```python
from build123d import *

# Parameters (mm, degrees)
SKETCH1_W                = 250
SKETCH1_H                = 100
BOSS_EXTRUDE1_DEPTH      = 4
SKETCH2_W                = 24
SKETCH2_H                = 4
BOSS_EXTRUDE2_DEPTH      = 4
SKETCH3_W                = 4
SKETCH3_H                = 40
SKETCH3_H_2              = 20
CUT_EXTRUDE1_DEPTH       = 5
M4_CLEARANCE_HOLE1_D     = 4.3
M4_CLEARANCE_HOLE1_DEPTH = 6
M4_CLEARANCE_HOLE1_TIP   = 1.291850331
CUT_EXTRUDE2_DEPTH       = 10
SKETCH7_W                = 13
SKETCH7_H                = 5
CUT_EXTRUDE3_DEPTH       = 10
CUT_EXTRUDE4_DEPTH       = 10


with BuildPart() as part:
    # Sketch1 → Boss-Extrude1 (new body)
    with BuildSketch(Plane.XY):
        Rectangle(SKETCH1_W, SKETCH1_H)
    extrude(amount=BOSS_EXTRUDE1_DEPTH)

    # Sketch2 → Boss-Extrude2 (add)
    with BuildSketch(Plane.XZ.offset(50)):
        with Locations((-78, 2)):
            Rectangle(SKETCH2_W, SKETCH2_H)
        with Locations((-42, 2)):
            Rectangle(SKETCH2_W, SKETCH2_H)
        with Locations((42, 2)):
            Rectangle(SKETCH2_W, SKETCH2_H)
        with Locations((78, 2)):
            Rectangle(SKETCH2_W, SKETCH2_H)
    boss_extrude2 = extrude(amount=BOSS_EXTRUDE2_DEPTH)

    # Sketch3 → Cut-Extrude1 (cut, through all)
    with BuildSketch(Plane.XY.offset(4)):
        with Locations((-8.5, 30)):
            Rectangle(SKETCH3_W, SKETCH3_H)
        with Locations((-8.5, -12)):
            Rectangle(SKETCH3_W, SKETCH3_H_2)
        with Locations((8.5, -12)):
            Rectangle(SKETCH3_W, SKETCH3_H_2)
        with Locations((8.5, 30)):
            Rectangle(SKETCH3_W, SKETCH3_H)
    extrude(amount=-CUT_EXTRUDE1_DEPTH, mode=Mode.SUBTRACT)

    # Mirror1: Boss-Extrude2 across plane
    add(boss_extrude2.mirror(Plane.ZX))

    # M4 Clearance Hole1
    with Locations(Plane.XY.offset(4)):
        with Locations((-8.5, 4), (8.5, 4)):
            Hole(M4_CLEARANCE_HOLE1_D / 2, depth=M4_CLEARANCE_HOLE1_DEPTH)
            with Locations((0, 0, -(M4_CLEARANCE_HOLE1_DEPTH + M4_CLEARANCE_HOLE1_TIP / 2))):  # 118° drill point
                Cone(0, M4_CLEARANCE_HOLE1_D / 2, M4_CLEARANCE_HOLE1_TIP, mode=Mode.SUBTRACT)

    # Sketch6 → Cut-Extrude2 (cut)
    with BuildSketch(Plane.XY.offset(4)):
        Polygon((-62.1, -50), (-57.9, -50), (-57.9, -40), (-55.5, -40), (-55.5, -39), (-56.25, -39), (-56.25, -36.5), (-57.9, -36.5), (-57.9, -33), (-62.1, -33), (-62.1, -36.5), (-63.75, -36.5), (-63.75, -39), (-64.5, -39), (-64.5, -40), (-62.1, -40), align=None)
        Polygon((57.9, -40), (57.9, -50), (62.1, -50), (62.1, -40), (64.5, -40), (64.5, -39), (63.75, -39), (63.75, -36.5), (62.1, -36.5), (62.1, -33), (57.9, -33), (57.9, -36.5), (56.25, -36.5), (56.25, -39), (55.5, -39), (55.5, -40), align=None)
        Polygon((62.1, 40), (62.1, 50), (57.9, 50), (57.9, 40), (55.5, 40), (55.5, 39), (56.25, 39), (56.25, 36.5), (57.9, 36.5), (57.9, 33), (62.1, 33), (62.1, 36.5), (63.75, 36.5), (63.75, 39), (64.5, 39), (64.5, 40), align=None)
        Polygon((-57.9, 50), (-62.1, 50), (-62.1, 40), (-64.5, 40), (-64.5, 39), (-63.75, 39), (-63.75, 36.5), (-62.1, 36.5), (-62.1, 33), (-57.9, 33), (-57.9, 36.5), (-56.25, 36.5), (-56.25, 39), (-55.5, 39), (-55.5, 40), (-57.9, 40), align=None)
    extrude(amount=-CUT_EXTRUDE2_DEPTH, mode=Mode.SUBTRACT)

    # Sketch7 → Cut-Extrude3 (cut)
    with BuildSketch(Plane.XY.offset(4)):
        with Locations((0, 47.5)):
            Rectangle(SKETCH7_W, SKETCH7_H)
    extrude(amount=-CUT_EXTRUDE3_DEPTH, mode=Mode.SUBTRACT)

    # Sketch8 → Cut-Extrude4 (cut)
    with BuildSketch(Plane.XY.offset(4)):
        Polygon((-15.5, 50), (-32.700401322, 262.698056725), (-161.835837728, 81.113354009), (-171.999440278, -88.149719236), (-15.5, -103.395123062), align=None)
    extrude(amount=-CUT_EXTRUDE4_DEPTH, mode=Mode.SUBTRACT)


solid = part.part
```
Geometry: final body of the model. Coordinates: model frame, mm. A direction names the side the tool comes from. Coordinates: 2 decimals unless noted, no trailing zeros. Order: outer loops, then holes, each group sorted by start corner. A loop starts at its lowest first (then second) coordinate and runs counter-clockwise, first axis right, second up. Notation, with made-up numbers: M 52.25,-30.5 L 69.25,-30.5 A21 ccw 69.25,4.5 Z; hole C 64,41.25 d4. An arc over 180 degrees is marked long. Answer in a Markdown table with one row per item. Add a question column.
Q1. Reachability of faces 1 (the flat face through (66, -52, 2)), 2 (the flat face through (7, -50, 2)), 3 (the flat face through (107, -50, 2)), 4 (the flat face through (107, 50, 2)), 5 (the flat face through (-6.5, 27, 2)) from +Z, -Z, +X, -X, +Y, -Y: full face, straight path, thin tool, end or side. Return the list, or none.
Q2. Section query B-B on y = 4. Return the cut outline in (x, z).
Q3. Section query A-A on x = -8.5. Return the cut outline in (y, z).
Q4. Mould query, pull axis Y, two halves, no side actions, for faces 6 (the flat face through (57.9, -35, 2)), 7 (the flat face through (0, 45, 2)), 8 (the flat face through (-10.5, -12, 2)). Classes: released by +Y, released by -Y, zero draft, split by the parting line, or undercut.
Q5. Section query C-C on y = -46. Return the cut outline in (x, z), and give its area (3 significant figures).
Q6. Contact query for flat-ended pins moving along their axis: P1, Ø1.2, axis at x = 8, z = 2.5, coming from the -Y side; P2, Ø1.5, axis at x = 7.5, y = 37.5, coming from the -Z side; P3, Ø0.5, axis at x = 63, z = 1, coming from the +Y side; P4, Ø2, axis at y = -51.5, z = 2, coming from the +X side. Output: stop coordinate, or through.
Q7. Section query D-D on z = 2.5. Count the separate pieces of the cut face and the enclosed holes in it, and give its area (3 significant figures).
Q8. Line query: L1, parallel to X at y = 22, z = 3.65; L2, parallel to X at y = 35, z = 3.1; L3, parallel to Y at x = -8.5, z = 2.15. Output: solid intervals per line, ascending.
Completed:
| question | item | result |
|---|---|---|
| 1 | face 1 | +Z, -Z, -Y |
| 1 | face 2 | +Z, -Z, -X, -Y |
| 1 | face 3 | +Z, -Z, +X, -Y |
| 1 | face 4 | +Z, -Z, +X, +Y |
| 1 | face 5 | +Z, -Z, +Y |
| 2 | outline | M -15.5,0 L -10.65,0 L -10.65,4 L -15.5,4 Z; M -6.35,0 L 6.35,0 L 6.35,4 L -6.35,4 Z; M 10.65,0 L 125,0 L 125,4 L 10.65,4 Z |
| 3 | outline | M -50,0 L -22,0 L -22,4 L -50,4 Z; M -2,0 L 1.85,0 L 1.85,4 L -2,4 Z; M 6.15,0 L 10,0 L 10,4 L 6.15,4 Z |
| 4 | face 6 | zero draft |
| 4 | face 7 | released by +Y |
| 4 | face 8 | undercut |
| 5 | outline | M -15.5,0 L 57.9,0 L 57.9,4 L -15.5,4 Z; M 62.1,0 L 125,0 L 125,4 L 62.1,4 Z |
| 5 | area | 545 mm2 |
| 6 | P1 | stops at y = -50 |
| 6 | P2 | passes through |
| 6 | P3 | stops at y = 50 |
| 6 | P4 | stops at x = 90 |
| 7 | separate pieces | 1 |
| 7 | enclosed holes | 4 |
| 7 | area | 13,700 mm2 |
| 8 | L1 | x = -15.5 to -10.5, -6.5 to 6.5, 10.5 to 125 |
| 8 | L2 | x = -15.5 to -10.5, -6.5 to 6.5, 10.5 to 57.9, 62.1 to 125 |
| 8 | L3 | y = -50 to -22, -2 to 1.85, 6.15 to 10 |
